Part print with two shaded views. Sizes in mm from the minimum x, y, z corner. A direction names the side the tool comes from. Coordinates: 2 decimals unless noted, no trailing zeros. Order: outer loops, then holes, each group sorted by start corner. A loop starts at its lowest first (then second) coordinate and runs counter-clockwise, first axis right, second up. Notation, with made-up numbers: M -37.75,14.25 L -27.75,14.25 A8 ccw -27.75,23.25 Z; hole C 63,-1.75 d5. An arc over 180 degrees is marked long. Answer in a Markdown table with one row per item. Add a question column.
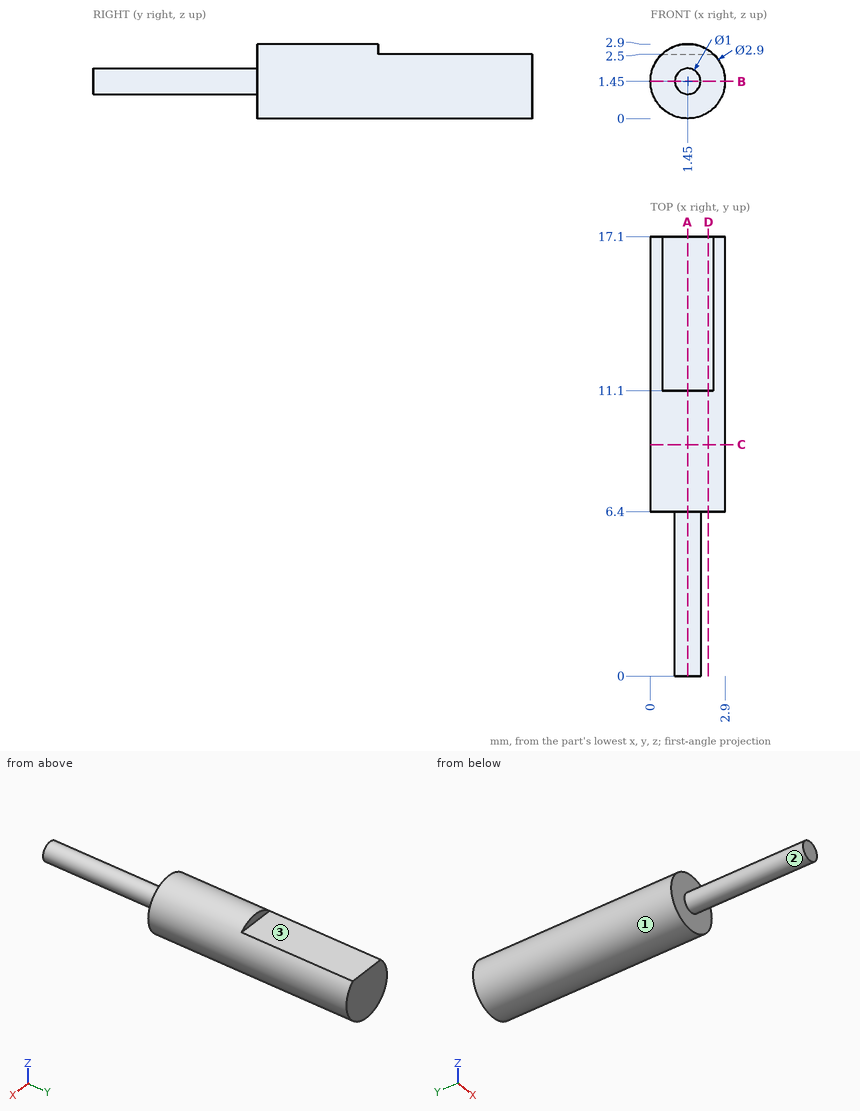
(1) Slice it at D-D (x = 2.25). List the corners of the cut face in (y, z), and give its area (3 significant figures).
(2) Wall check: line 1 (Y direction, x = 2.2, z = 0.4); line 2 (X direction, y = 4.5, z = 1.5); line 3 (Y direction, x = 0.75, z = 2.6). Give the ranges that are in metal, low to high.
(3) Slice it at B-B (z = 1.45). List the corners of the cut face in (x, y).
(4) Slice it at A-A (x = 1.45). List the corners of the cut face in (y, z), and give its area (3 significant figures).
(5) Slice it at C-C (y = 9). List the corners of the cut face in (x, z).
(6) Drop flat-ended pins along their axis: P1, Ø1.4, axis at x = 2, z = 1, coming from the -Y side; P2, Ø0.6, axis at x = 1.5, y = 15.5, coming from the +Z side. Give the stop position or say it passes through.
(7) 3-axis set-ups, long thin cutter, end or side, ignore diameter. For the marked faces 1, 2 and 3: which of +Z, -Z, +X, -X, +Y, -Y reach the whole face in a straight line?
Computed:
| question | item | result |
|---|---|---|
| 1 | outline | M 6.4,0.24 L 17.1,0.24 L 17.1,2.5 L 11.1,2.5 L 11.1,2.66 L 6.4,2.66 Z |
| 1 | area | 24.9 mm^2 |
| 2 | line 1 | y = 6.4 to 17.1 |
| 2 | line 2 | x = 0.95 to 1.95 |
| 2 | line 3 | y = 6.4 to 11.1 |
| 3 | outline | M 0,6.4 L 0.95,6.4 L 0.95,0 L 1.95,0 L 1.95,6.4 L 2.9,6.4 L 2.9,17.1 L 0,17.1 Z |
| 4 | outline | M 0,0.95 L 6.4,0.95 L 6.4,0 L 17.1,0 L 17.1,2.5 L 11.1,2.5 L 11.1,2.9 L 6.4,2.9 L 6.4,1.95 L 0,1.95 Z |
| 4 | area | 35.0 mm^2 |
| 5 | outline | C 1.45,1.45 d2.9 |
| 6 | P1 | stops at y = 0 |
| 6 | P2 | stops at z = 2.5 |
| 7 | face 1 | +Y, -Y |
| 7 | face 2 | -Y |
| 7 | face 3 | +Z, +X, -X, +Y |
